```python
from build123d import *

# Parameters (mm, degrees)
CROQUIS1_W              = 34
CROQUIS1_H              = 20
CROQUIS1_R              = 1.5
BASE_DEPTH              = 2
SALIENTE_EXTRUIR2_DEPTH = 20
REDONDEO1_R             = 0.5


with BuildPart() as part:
    # Croquis1 → Base (new body)
    with BuildSketch(Plane.XY):
        Rectangle(CROQUIS1_W, CROQUIS1_H)
        with Locations((12.5, 5)):
            Circle(CROQUIS1_R, mode=Mode.SUBTRACT)
        with Locations((-12.5, 5)):
            Circle(CROQUIS1_R, mode=Mode.SUBTRACT)
        with Locations((-12.5, -5)):
            Circle(CROQUIS1_R, mode=Mode.SUBTRACT)
        with Locations((12.5, -5)):
            Circle(CROQUIS1_R, mode=Mode.SUBTRACT)
    extrude(amount=BASE_DEPTH)

    # Croquis2 → Saliente-Extruir2 (add, through all)
    with BuildSketch(Plane(origin=(0, 10, 0), x_dir=(1, 0, 0), z_dir=(0, 1, 0))):
        Polygon((-5, 0), (-6.5, 0), (-6.5, 4.8), (-3, 4.8), (-3, 3.741089378), (-4.040563392, 2.3), (-4.040563392, 3.482732018), (-5, 3.482732018), align=None)
        Polygon((3, 4.8), (6.5, 4.8), (6.5, 0), (5, 0), (5, 3.482732018), (4.040563392, 3.482732018), (4.040563392, 2.3), (3, 3.741089378), align=None)
    extrude(amount=-SALIENTE_EXTRUIR2_DEPTH)

    # Redondeo1
    redondeo1_edges = [part.edges().sort_by_distance(p)[0] for p in [
        (-6.5, 0, 0),
        (6.5, 0, 0),
    ]]
    fillet(redondeo1_edges, radius=REDONDEO1_R)


solid = part.part
```
Design review of the part built by this model. Coordinates are the model's own, in mm. A direction names the side the tool comes from. Coordinates: 2 decimals unless noted, no trailing zeros. Loops run counter-clockwise (first coordinate to the right, second up) from the corner with the lowest first, then second, coordinate; pieces in that order, holes last. Notation, with made-up numbers: (-20.5, -9) - (34.5, -9) arc R23 ccw to (34.5, 26) - close; hole circle Ø10 at (-36, -20). An arc over 180 degrees is marked (long way). Use CSV: the item, a comma, the result in double quotes. Start each with the question number.
1) For pin 1 Ø1.3 at (y, z) = (-5, -3) entering from +X; pin 2 Ø0.6 at (y, z) = (5, -2.5) entering from -X; pin 3 Ø5 at (x, y) = (12, -4) entering from -Z, all flat-tipped, find the tip position at first contact; note any pin that passes through.
2) The part is to be moulded in two halves that separate along Z. For faces 1 (the flat face through (5, 0, -4.8)), 2 (the flat face through (-17, 0, 1)), 3 (the flat face through (-4.5, 0.1, -3.483)), say which applies: +Z half, -Z half, draft (parallel to the pull), parting line (faces both ways), or undercut.
3) Consider section C-C on x = -12.5. Write out the cut boundary in (y, z), then the cut area to 3 significant figures.
4) Consider section A-A on y = 5. Give the number of separate pieces and of enclosed holes in the cut face, then the cut area to 3 significant figures.
5) Consider section B-B on z = -1.75. Write out the cut boundary in (x, y), then the cut area to 3 significant figures.
6) Wall thickness on L1, parallel to Y at x = -12.5, z = 1.2; L2, parallel to X at y = 1.5, z = -1.5; L3, parallel to X at y = 4, z = -3.25: over which ranges is each line inside the solid? List them lowest first. Write a range as from..to.
7) Tool access review of faces 4 (the flat face through (-6.5, 0, -3)), 5 (the flat face through (-3, 0, -4)), 6 (the flat face through (5, 0, -2)): name each direction out of +Z, -Z, +X, -X, +Y, -Y from which nothing blocks a thin tool from reaching the whole face with its end or side.
8) Consider section D-D on y = 3. Write out the cut boundary in (x, z), then the cut area to 3 significant figures.
Geometry says:
1,pin 1,"x = 6.5"
1,pin 2,"x = -6.5"
1,pin 3,"z = 0"
2,face 1,"-Z half"
2,face 2,"draft"
2,face 3,"undercut"
3,outline,"(-10, 0) - (-6.5, 0) - (-6.5, 2) - (-10, 2) - close; (-3.5, 0) - (3.5, 0) - (3.5, 2) - (-3.5, 2) - close; (6.5, 0) - (10, 0) - (10, 2) - (6.5, 2) - close"
3,area,"28.0 mm^2"
4,separate pieces,"3"
4,enclosed holes,"0"
4,area,"76.7 mm^2"
5,outline,"(-6.5, -10) - (-5, -10) - (-5, 10) - (-6.5, 10) - close; (5, -10) - (6.5, -10) - (6.5, 10) - (5, 10) - close"
5,area,"60.0 mm^2"
6,L1,"-10..-6.5, -3.5..3.5, 6.5..10"
6,L2,"-6.5..-5, 5..6.5"
6,L3,"-6.5..-5, -4.04..-3.35, 3.35..4.04, 5..6.5"
7,face 4,"-Z, -X, +Y, -Y"
7,face 5,"-Z, +Y, -Y"
7,face 6,"+Y, -Y"
8,outline,"(-17, 0) - (-7, 0) arc R0.5 cw to (-6.5, -0.5) - (-6.5, -4.8) - (-3, -4.8) - (-3, -3.74) - (-4.04, -2.3) - (-4.04, -3.48) - (-5, -3.48) - (-5, 0) - (5, 0) - (5, -3.48) - (4.04, -3.48) - (4.04, -2.3) - (3, -3.74) - (3, -4.8) - (6.5, -4.8) - (6.5, -0.5) arc R0.5 cw to (7, 0) - (17, 0) - (17, 2) - (-17, 2) - close"
8,area,"88.7 mm^2"
